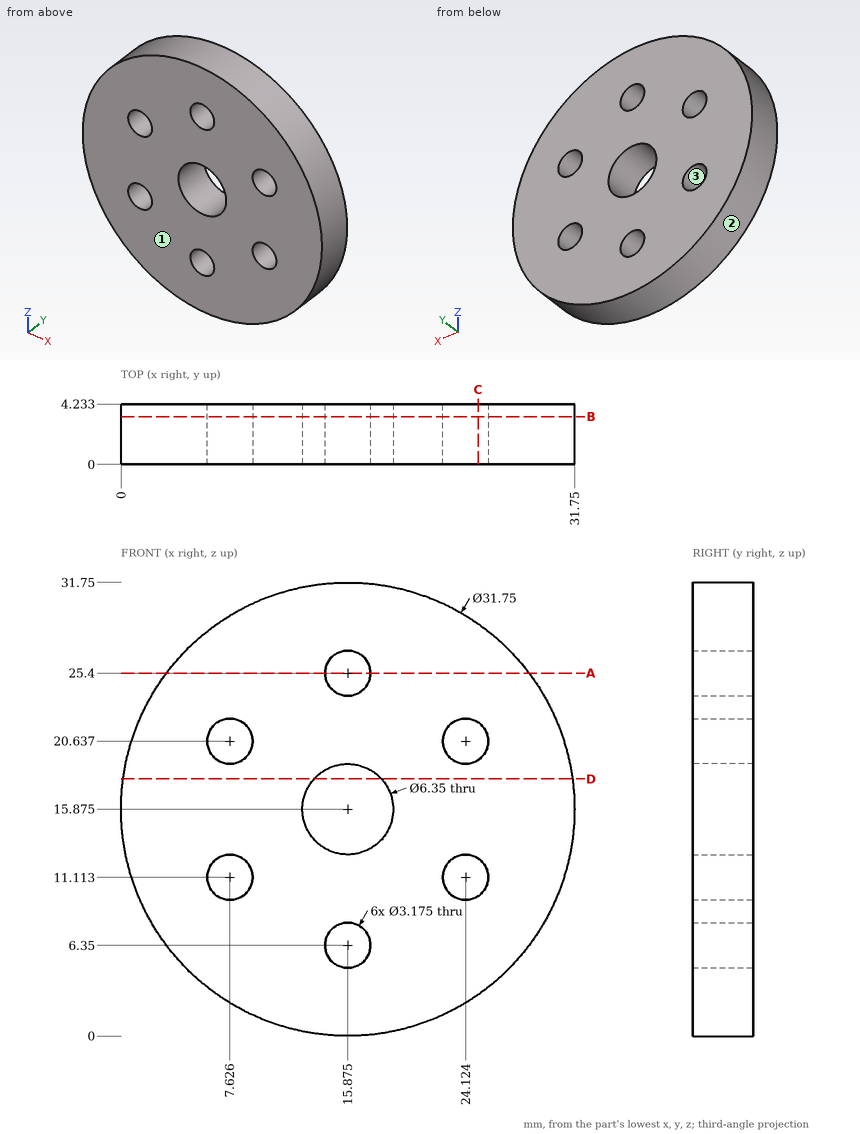
Design review of the part shown in the three views and the two pictorial views. Dimensions are in mm from the part's minimum x, y and z. Round coordinates to 2 decimals unless told otherwise and drop trailing zeros. Write each loop counter-clockwise with the first axis right and the second up, starting at its lowest first coordinate (ties: lowest second). Pieces come first, ordered by that corner, then holes.
Item 1: Consider section B-B on y = 3.35. Count the separate pieces of the cut face and the enclosed holes in it.
Item 2: For pin 1 Ø2.5 at (x, z) = (15.875, 6.35) entering from +Y; pin 2 Ø1 at (x, y) = (5.5, 2.5) entering from -Z (1 decimal); pin 3 Ø1 at (y, z) = (3.5, 27) entering from +X, all flat-tipped, find the tip position at first contact; note any pin that passes through.
Item 3: Consider section C-C on x = 25. Give the boundary of the cut face in (y, z) (1 decimal).
Item 4: Draft analysis for pull direction Z (two halves, no side actions). For the marked faces 1, 2 and 3, state which applies: released by +Z, released by -Z, zero draft, split by the parting line, or undercut.
Item 5: Wall thickness on L1, parallel to Z at x = 8, y = 1.2 (1 decimal); L2, parallel to Z at x = 24, y = 1.55 (1 decimal); L3, parallel to X at y = 2.5, z = 14.5 (1 decimal): over which ranges is each line inside the solid? List them lowest first.
Item 6: Consider section A-A on z = 25.4. Give the boundary of the cut face in (x, y) (1 decimal).
Item 7: Consider section D-D on z = 18. Give the boundary of the cut face in (x, y) (1 decimal), and give its area (3 significant figures).
Check values:
1. separate pieces: 1
1. enclosed holes: 7
2. pin 1: passes through
2. pin 2: stops at z = 3.4
2. pin 3: stops at x = 27.67
3. outline: (0, 2.9) - (4.2, 2.9) - (4.2, 9.8) - (0, 9.8) - close; (0, 12.4) - (4.2, 12.4) - (4.2, 19.3) - (0, 19.3) - close; (0, 22) - (4.2, 22) - (4.2, 28.9) - (0, 28.9) - close
4. face 1: zero draft
4. face 2: split by the parting line
4. face 3: undercut
5. L1: z = 2.1 to 9.6, 12.7 to 19.1, 22.2 to 29.7
5. L2: z = 2.2 to 9.5, 12.7 to 19.1, 22.2 to 29.5
5. L3: x = 0.1 to 13, 18.7 to 31.7
6. outline: (3.2, 0) - (14.3, 0) - (14.3, 4.2) - (3.2, 4.2) - close; (17.5, 0) - (28.6, 0) - (28.6, 4.2) - (17.5, 4.2) - close
7. outline: (0.1, 0) - (13.5, 0) - (13.5, 4.2) - (0.1, 4.2) - close; (18.2, 0) - (31.6, 0) - (31.6, 4.2) - (18.2, 4.2) - close
7. area: 113 mm2
